Part model, mm, in its own coordinate system. A direction names the side the tool comes from. Round coordinates to 2 decimals unless told otherwise and drop trailing zeros. Write each loop counter-clockwise with the first axis right and the second up, starting at its lowest first coordinate (ties: lowest second). Pieces come first, ordered by that corner, then holes. Notation, with made-up numbers: M -36,73.5 L -14,73.5 A33 cw -14,104.5 Z; hole C 49,49.25 d5. An arc over 180 degrees is marked long. Answer as a JSON object with one key per item and string values. Group by question number.
1. Which spindle directions (+Z, -Z, +X, -X, +Y, -Y) get a long thin tool onto all of the face, cutting with end or side? Do faces 5 (the face through (48.75, 7, 5)), 6 (the face through (-32.377, 18.302, 7.056)). Say none if no direction does.
2. Two-plate mould, pull along X, no slides. Class faces 1 (the face through (41, 14, 3)), 2 (the face through (-35.5, 13.9, 3)), 3 (the face through (-48.18, 23.4, 5.58)), 4 (the face through (-1, -10.5, 5)): +X half, -X half, draft (parallel to the pull), parting line (faces both ways), or undercut.
3. Band-saw the part on C-C, the plane z = 7.75. Write the cut outline in (x, y).
4. Band-saw the part on B-B, the plane x = -38.1. Write the cut outline in (y, z).
5. Band-saw the part on D-D, the plane z = 1.25. Write the cut outline in (x, y), plus the area to 3 significant figures.
6. Drop a flat-ended pin along its axis: pin 1 (7 mm diameter, centred on x = -38.1, y = 16.5, fed in from +Z). Give the stop position or say it passes through.
7. Band-saw the part on A-A, the plane y = 4.05. Write the cut outline in (x, z), plus the area to 3 significant figures.
8. Drill centre lines: line 1 (X direction, y = 4, z = 5.25); line 2 (X direction, y = 14, z = 2.75); line 3 (Y direction, x = -43, z = 2.5). Where is each one in solid material? Low to high. Write a range as from..to.
from build123d import *

# Parameters (mm, degrees)
F0_W     = 97.5
F0_H     = 34.5
F0_R     = 1.7
F0_R_2   = 3.4
F1_DEPTH = 11
F2_R     = 6
F3_DEPTH = 8
F4_R     = 2


with BuildPart() as f1:
    # F0 (on Top) → F1 (new body)
    with BuildSketch(Plane.XY):
        with Locations((0, 6.75)):
            Rectangle(F0_W, F0_H)
        with Locations((-43.65, -4.05)):
            Circle(F0_R, mode=Mode.SUBTRACT)
        with Locations((-43.65, 4.05)):
            Circle(F0_R, mode=Mode.SUBTRACT)
        with Locations((43.65, -4.05)):
            Circle(F0_R, mode=Mode.SUBTRACT)
        with Locations((43.65, 4.05)):
            Circle(F0_R, mode=Mode.SUBTRACT)
        with Locations((-38.1, 16.5)):
            Circle(F0_R_2, mode=Mode.SUBTRACT)
        with Locations((38.1, 16.5)):
            Circle(F0_R_2, mode=Mode.SUBTRACT)
    extrude(amount=F1_DEPTH)

    # F2 (on face) → F3 (cut)
    with BuildSketch(Plane.XY.offset(11)):
        with Locations((-38.1, 16.5)):
            Circle(F2_R)
        with Locations((38.1, 16.5)):
            Circle(F2_R)
    extrude(amount=-F3_DEPTH, mode=Mode.SUBTRACT)

    # F4
    f4_edges = [f1.edges().sort_by_distance(p)[0] for p in [
        (-48.75, -10.5, 5.5),
        (-48.75, 24, 5.5),
        (48.75, -10.5, 5.5),
        (48.75, 24, 5.5),
    ]]
    fillet(f4_edges, radius=F4_R)


solid = f1.part
Worked answers:
{
 "1": {"face 5": "+Z, -Z, +X, +Y, -Y", "face 6": "+Z"},
 "2": {"face 1": "undercut", "face 2": "undercut", "face 3": "-X half", "face 4": "draft"},
 "3": {"outline": "M -48.75,-8.5 A2 ccw -46.75,-10.5 L 46.75,-10.5 A2 ccw 48.75,-8.5 L 48.75,22 A2 ccw 46.75,24 L -46.75,24 A2 ccw -48.75,22 Z; hole C -43.65,-4.05 d3.4; hole C -43.65,4.05 d3.4; hole C -38.1,16.5 d12; hole C 38.1,16.5 d12; hole C 43.65,-4.05 d3.4; hole C 43.65,4.05 d3.4"},
 "4": {"outline": "M -10.5,0 L 13.1,0 L 13.1,3 L 10.5,3 L 10.5,11 L -10.5,11 Z; M 19.9,0 L 24,0 L 24,11 L 22.5,11 L 22.5,3 L 19.9,3 Z"},
 "5": {"outline": "M -48.75,-8.5 A2 ccw -46.75,-10.5 L 46.75,-10.5 A2 ccw 48.75,-8.5 L 48.75,22 A2 ccw 46.75,24 L -46.75,24 A2 ccw -48.75,22 Z; hole C -43.65,-4.05 d3.4; hole C -43.65,4.05 d3.4; hole C -38.1,16.5 d6.8; hole C 38.1,16.5 d6.8; hole C 43.65,-4.05 d3.4; hole C 43.65,4.05 d3.4", "area": "3,250 mm^2"},
 "6": {"pin 1": "stops at z = 3"},
 "7": {"outline": "M -48.75,0 L -45.35,0 L -45.35,11 L -48.75,11 Z; M -41.95,0 L 41.95,0 L 41.95,11 L -41.95,11 Z; M 45.35,0 L 48.75,0 L 48.75,11 L 45.35,11 Z", "area": "998 mm^2"},
 "8": {"line 1": "x = -48.75..-45.35, -41.95..41.95, 45.35..48.75", "line 2": "x = -48.75..-40.4, -35.8..35.8, 40.4..48.75", "line 3": "y = -10.5..-5.62, -2.48..2.48, 5.62..24"}
}
